from build123d import *

# Parameters (mm, degrees)
BOSS_EXTRUDE1_DEPTH         = 227.5
TAP_DRILL_FOR_M5X0_8_TAP1_D = 5
F_5_0_5_DIAMETER_HOLE1_D    = 5


with BuildPart() as part:
    # Sketch1 → Boss-Extrude1 (new body)
    with BuildSketch(Plane.XY):
        Polygon((0, 5), (0, 0), (5, 0), (20, 0), (20, 5), (5, 5), (5, 20), (0, 20), align=None)
    extrude(amount=BOSS_EXTRUDE1_DEPTH)

    # Tap Drill for M5x0.8 Tap1 (through all)
    with Locations(Plane(origin=(0, 5, 0), x_dir=(1, 0, 0), z_dir=(0, 1, 0))):
        with Locations((12.5, -203.75), (12.5, -143.75), (12.5, -83.75), (12.5, -23.75)):
            Hole(TAP_DRILL_FOR_M5X0_8_TAP1_D / 2)

    # Ø5.0 (5) Diameter Hole1 (through all)
    with Locations(Plane(origin=(5, 0, 0), x_dir=(0, 0, -1), z_dir=(1, 0, 0))):
        with Locations((-177.5, 12.346163158), (-132.5, 12.346163158), (-95, 12.346163158), (-50, 12.346163158)):
            Hole(F_5_0_5_DIAMETER_HOLE1_D / 2)


solid = part.part
Work out the finished part from the listing and answer in its coordinate system (mm). A direction names the side the tool comes from. Give positions to 0.01 mm unless a question says otherwise; leave off trailing zeros. Loops run counter-clockwise (first coordinate to the right, second up) from the corner with the lowest first, then second, coordinate; pieces in that order, holes last. Notation, with made-up numbers: (68.5, 66.5) -> (105.5, 66.5) arc R20 ccw to (105.5, 87.5) -> close; hole circle Ø7 at (-33, 47.25). An arc over 180 degrees is marked (long way). Use a Markdown table: item, result. Add a question column.
1) The part is cut by section A-A, the plane z = 177.5. Determine the outline of the cut face in (x, y).
2) Which of the six approach directions +Z, -Z, +X, -X, +Y, -Y give full straight-line access (tool end or side, diameter ignored) to faces 4 (the cylindrical face through (12.83, 2.47, 201.27)), 5 (the flat face through (5, 12, 112))?
3) The part is cut by section B-B, the plane x = 12.5. Determine the outline of the cut face in (y, z), plus the area to 3 significant figures.
4) For a pull along X with two mould halves and no side action, classify faces 1 (the cylindrical face through (2.465, 13.097, 179.885)), 2 (the cylindrical face through (14.998, 2.465, 83.64)), 3 (the flat face through (0, 10, 112)) as +X half, -X half, draft (parallel to the pull), parting line (faces both ways), or undercut.
5) Each of these flat-tipped pins is pushed along its axis until it touches: P1, Ø12, axis at x = 15, z = 83.5, coming from the +Y side; P2, Ø3, axis at y = 12.35, z = 132.5, coming from the +X side; P3, Ø4.5, axis at y = 10.5, z = 94.5, coming from the +X side. Where does it stop, or does it pass through?
6) Consider line 1 along Z through (x, y) = (12.5, 1); line 2 along X through (y, z) = (2.85, 23.75); line 3 along Y through (x, z) = (2.95, 132.5). Determine where each line is inside the solid, lowest interval first.
7) The part is cut by section D-D, the plane z = 111.5. Determine the outline of the cut face in (x, y), plus the area to 3 significant figures.
8) The part is cut by section C-C, the plane y = 3. Determine the outline of the cut face in (x, z).
Reported:
| question | item | result |
|---|---|---|
| 1 | outline | (0, 0) -> (20, 0) -> (20, 5) -> (5, 5) -> (5, 9.85) -> (0, 9.85) -> close; (0, 14.85) -> (5, 14.85) -> (5, 20) -> (0, 20) -> close |
| 2 | face 4 | +Y, -Y |
| 2 | face 5 | +Z, -Z, +X, +Y |
| 3 | outline | (0, 0) -> (5, 0) -> (5, 21.25) -> (0, 21.25) -> close; (0, 26.25) -> (5, 26.25) -> (5, 81.25) -> (0, 81.25) -> close; (0, 86.25) -> (5, 86.25) -> (5, 141.25) -> (0, 141.25) -> close; (0, 146.25) -> (5, 146.25) -> (5, 201.25) -> (0, 201.25) -> close; (0, 206.25) -> (5, 206.25) -> (5, 227.5) -> (0, 227.5) -> close |
| 3 | area | 1,040 mm^2 |
| 4 | face 1 | draft |
| 4 | face 2 | undercut |
| 4 | face 3 | -X half |
| 5 | P1 | stops at y = 5 |
| 5 | P2 | passes through |
| 5 | P3 | stops at x = 5 |
| 6 | line 1 | z = 0 to 21.25, 26.25 to 81.25, 86.25 to 141.25, 146.25 to 201.25, 206.25 to 227.5 |
| 6 | line 2 | x = 0 to 10, 15 to 20 |
| 6 | line 3 | y = 0 to 9.85, 14.85 to 20 |
| 7 | outline | (0, 0) -> (20, 0) -> (20, 5) -> (5, 5) -> (5, 20) -> (0, 20) -> close |
| 7 | area | 175 mm^2 |
| 8 | outline | (0, 0) -> (20, 0) -> (20, 227.5) -> (0, 227.5) -> close; hole circle Ø5 at (12.5, 23.75); hole circle Ø5 at (12.5, 83.75); hole circle Ø5 at (12.5, 143.75); hole circle Ø5 at (12.5, 203.75) |
